Geometry: final body of the model. Coordinates: model frame, mm. Face numbers are marked on the shaded views. A direction names the side the tool comes from. Round coordinates to 2 decimals unless told otherwise and drop trailing zeros. Write each loop counter-clockwise with the first axis right and the second up, starting at its lowest first coordinate (ties: lowest second). Pieces come first, ordered by that corner, then holes. Notation, with made-up numbers: (-20.75, 31) -> (-8.75, 31) arc R17 ccw to (-8.75, 50) -> close; hole circle Ø9 at (63.5, -37). An arc over 180 degrees is marked (long way). One line per item, written item: value. Start each with the question number.
from build123d import *

# Parameters (mm, degrees)
SKETCH1_W            = 12.65
SKETCH1_H            = 5.1
BOSS_EXTRUDE1_DEPTH  = 5.4
SKETCH2_W            = 11.25
SKETCH2_H            = 3.7
CUT_EXTRUDE1_DEPTH   = 3.5
CUT_EXTRUDE2_REACH   = 11.756
SKETCH3_W            = 2.35
SKETCH3_H            = 3.5
CUT_EXTRUDE5_REACH   = 10.699
SKETCH4_W            = 0.4
SKETCH4_H            = 0.4
LPATTERN1_COUNT      = 5
LPATTERN1_PITCH      = 1.27
LPATTERN1_COUNT_DIR2 = 2
LPATTERN1_PITCH_DIR2 = 1.27


with BuildPart() as part:
    # Sketch1 → Boss-Extrude1 (new body)
    with BuildSketch(Plane(origin=(0, 0, 0), x_dir=(1, 0, 0), z_dir=(0, 1, 0))):
        Rectangle(SKETCH1_W, SKETCH1_H)
    extrude(amount=BOSS_EXTRUDE1_DEPTH)

    # Sketch2 → Cut-Extrude1 (cut)
    with BuildSketch(Plane(origin=(0, 5.4, 0), x_dir=(1, 0, 0), z_dir=(0, 1, 0))):
        Rectangle(SKETCH2_W, SKETCH2_H)
    extrude(amount=-CUT_EXTRUDE1_DEPTH, mode=Mode.SUBTRACT)

    # Sketch3 → Cut-Extrude2 (cut, up to next)
    with BuildSketch(Plane.XY.offset(2.55), mode=Mode.PRIVATE) as cut_extrude2_sk1:
        with Locations((0, 3.65)):
            Rectangle(SKETCH3_W, SKETCH3_H)
    cut_extrude2_tool1 = extrude(cut_extrude2_sk1.sketch, amount=-CUT_EXTRUDE2_REACH, mode=Mode.PRIVATE) & part.part
    add(cut_extrude2_tool1.solids().sort_by_distance((0, 3.65, 2.55))[0], mode=Mode.SUBTRACT)

    # Sketch4 → Cut-Extrude5 (cut, up to next)
    with BuildSketch(Plane.XZ, mode=Mode.PRIVATE) as cut_extrude5_sk1:
        with Locations((-2.54, 0.635)):
            Rectangle(SKETCH4_W, SKETCH4_H)
    cut_extrude5_tool1 = extrude(cut_extrude5_sk1.sketch, amount=-CUT_EXTRUDE5_REACH, mode=Mode.PRIVATE) & part.part
    cut_extrude5 = cut_extrude5_tool1.solids().sort_by_distance((-2.54, 0, 0.635))[0]
    add(cut_extrude5, mode=Mode.SUBTRACT)

    # LPattern1: Cut-Extrude5 5 × 2
    with Locations(*[(i * LPATTERN1_PITCH, 0, -j * LPATTERN1_PITCH_DIR2) for i in range(LPATTERN1_COUNT) for j in range(LPATTERN1_COUNT_DIR2) if (i, j) != (0, 0)]):
        add(cut_extrude5, mode=Mode.SUBTRACT)


solid = part.part
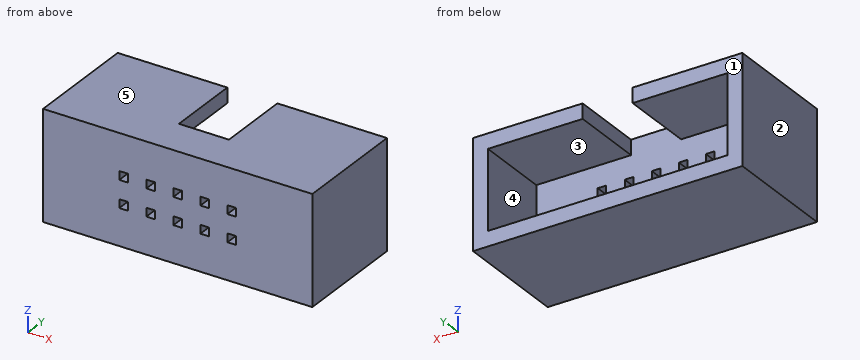
(1) Set-up query: the marked faces 4 and 5. Return all of +Z, -Z, +X, -X, +Y, -Y with unobstructed straight access to the full face (end or side cutting, diameter ignored); none if empty.
(2) Section query D-D (y = 1.45). Count the separate pieces of the cut face and the enclosed holes in it, and give its area (3 significant figures).
(3) Section query B-B (z = 2). Output: boundary loops of the cut face in (x, y) (3 decimals), and give its area (3 significant figures).
(4) Section query C-C (x = 4.5). Output: boundary loops of the cut face in (y, z), and give its area (3 significant figures).
(5) Section query A-A (y = 3.25). Output: boundary loops of the cut face in (x, z) (3 decimals), and give its area (3 significant figures).
(6) Pull-direction query (X, two-part tool) for the marked faces 1, 2 and 3; classes: pulls with the +X half, pulls with the -X half, needs draft (parallel to the pull), parting line crosses it, or undercut.
(7) Line query: probe 1 along Z at (x, y) = (-2.5, 0.4) (3 decimals); probe 2 along X at (y, z) = (1.4, -0.7) (3 decimals); probe 3 along Z at (x, y) = (2.5, 2.95). Output: solid intervals per line, ascending.
Results list:
1. face 4: +Y
1. face 5: +Z, +X, -X, +Y, -Y
2. separate pieces: 1
2. enclosed holes: 10
2. area: 62.9 mm^2
3. outline: (-6.325, 0) -> (6.325, 0) -> (6.325, 5.4) -> (1.175, 5.4) -> (1.175, 1.9) -> (-1.175, 1.9) -> (-1.175, 5.4) -> (-6.325, 5.4) -> close
3. area: 60.1 mm^2
4. outline: (0, -2.55) -> (5.4, -2.55) -> (5.4, -1.85) -> (1.9, -1.85) -> (1.9, 1.85) -> (5.4, 1.85) -> (5.4, 2.55) -> (0, 2.55) -> close
4. area: 14.6 mm^2
5. outline: (-6.325, -2.55) -> (6.325, -2.55) -> (6.325, 2.55) -> (1.175, 2.55) -> (1.175, 1.85) -> (5.625, 1.85) -> (5.625, -1.85) -> (-5.625, -1.85) -> (-5.625, 1.85) -> (-1.175, 1.85) -> (-1.175, 2.55) -> (-6.325, 2.55) -> close
5. area: 21.2 mm^2
6. face 1: needs draft
6. face 2: pulls with the -X half
6. face 3: undercut
7. probe 1: z = -2.55 to -0.835, -0.435 to 0.435, 0.835 to 2.55
7. probe 2: x = -6.325 to -2.74, -2.34 to -1.47, -1.07 to -0.2, 0.2 to 1.07, 1.47 to 2.34, 2.74 to 6.325
7. probe 3: z = -2.55 to -1.85, 1.85 to 2.55
